For this review, take the finished solid that the model builds, in its own axes (mm). A direction names the side the tool comes from. Coordinates: 2 decimals unless noted, no trailing zeros. Write each loop counter-clockwise with the first axis right and the second up, starting at its lowest first coordinate (ties: lowest second). Pieces come first, ordered by that corner, then holes. Notation, with made-up numbers: M -12.5,28 L 14.5,28 A28 ccw 14.5,67 Z; hole C 10.5,-23 d1. An arc over 180 degrees is marked long. One line per question, with ' | ' between items.
from build123d import *

# Parameters (mm, degrees)
F0_W         = 45.3698039055
F0_H         = 13.4970545769
F1_DEPTH     = 12.7
F2_T         = -2.54
F3_T1_DEPTH  = 40.2898039055
F4_T4_DEPTH  = 35.494099833
F4_T10_DEPTH = 35.494099833


# Not quite as in the source:
# - a fillet or chamfer that OpenCascade refuses, or shapes differently, is made with other operations: its cross-section is extruded or revolved along the edge and cut away or added


with BuildPart() as f1:
    # F0 (on Top) → F1 (new body)
    with BuildSketch(Plane.XY):
        with Locations((22.6849019527, -6.7485272884)):
            Rectangle(F0_W, F0_H)
    extrude(amount=F1_DEPTH)

    # F2
    f2_openings = [f1.faces().sort_by_distance(p)[0] for p in [
        (22.684902, -6.748527, 12.7),
    ]]
    offset(amount=F2_T, openings=f2_openings)

    # F3: chamfer of 5.08 on 2 edges, made by hand

    # F3_s2 → F3_t1 (cut)
    with BuildSketch(Plane.YZ.offset(2.54)):
        Polygon((-16.0370545769, 12.7), (-10.9570545769, 7.62), (-10.9570545769, 12.7), align=None)
        Polygon((2.54, 12.7), (-2.54, 7.62), (-2.54, 12.7), align=None)
    extrude(amount=F3_T1_DEPTH, mode=Mode.SUBTRACT)

    # F4: fillet of radius 5.08 on 2 edges, made by hand


with BuildPart() as f4_tool2:
    # F4_s3 → F4_t4 (new body)
    with BuildSketch(Plane.XZ.offset(24.4955772049)):
        with BuildLine():
            ThreePointArc((45.3698039055, 12.7), (43.5103948543, 10.8405909488), (42.8298039055, 8.3005909488))
            Line((42.8298039055, 8.3005909488), (42.8298039055, 12.7))
            Line((42.8298039055, 12.7), (45.3698039055, 12.7))
        make_face()
    extrude(amount=-F4_T4_DEPTH)

    split(bisect_by=Plane(origin=(0, -1.6685272884, -1.6685272884), x_dir=(1, 0, 0), z_dir=(0, 0.7071067812, 0.7071067812)), keep=Keep.TOP)

    split(bisect_by=Plane(origin=(0, -5.08, 5.08), x_dir=(1, 0, 0), z_dir=(0, -0.7071067812, 0.7071067812)), keep=Keep.TOP)


with BuildPart() as f1_1:
    add(f1.part)

    # F4_t1: cut F4_tool2
    add(f4_tool2.part, mode=Mode.SUBTRACT)


with BuildPart() as f4_tool8:
    # F4_s9 → F4_t10 (new body)
    with BuildSketch(Plane.XZ.offset(24.4955772049)):
        with BuildLine():
            ThreePointArc((2.54, 8.3005909488), (1.8594090512, 10.8405909488), (0, 12.7))
            Line((0, 12.7), (2.54, 12.7))
            Line((2.54, 12.7), (2.54, 8.3005909488))
        make_face()
    extrude(amount=-F4_T10_DEPTH)

    split(bisect_by=Plane(origin=(0, -1.6685272884, -1.6685272884), x_dir=(1, 0, 0), z_dir=(0, 0.7071067812, 0.7071067812)), keep=Keep.TOP)

    split(bisect_by=Plane(origin=(0, -5.08, 5.08), x_dir=(1, 0, 0), z_dir=(0, -0.7071067812, 0.7071067812)), keep=Keep.TOP)


with BuildPart() as f1_2:
    add(f1_1.part)

    # F4_t7: cut F4_tool8
    add(f4_tool8.part, mode=Mode.SUBTRACT)


solid = f1_2.part
1) We need section B-B on x = 20.5. State the section outline as (y, z) points.
Responses:
outline: M -13.5,0 L 0,0 L 0,10.16 L -2.54,7.62 L -2.54,2.54 L -10.96,2.54 L -10.96,7.62 L -13.5,10.16 Z
2) To check wall thickness, follow line 1 along Y through (x, z) = (32, 7); line 2 along Z through (x, y) = (39, -10); line 3 along X through (y, z) = (-8.75, 4.75). State the ranges of each line that lie inside material, in increasing order. Write a range as [from, to].
Responses:
line 1: [-13.5, -10.96], [-2.54, 0] | line 2: [0, 2.54] | line 3: [0, 2.54], [42.83, 45.37]
3) We need section C-C on z = 10.75. State the section outline as (x, y) points, then the cut area to 3 significant figures.
Responses:
outline: M 0,-13.5 L 1.91,-13.5 L 1.91,0 L 0,0 Z; M 43.46,-13.5 L 45.37,-13.5 L 45.37,0 L 43.46,0 Z | area: 51.6 mm^2
4) Machinability: for faces 1 (the flat face through (2.54, -7, 5)), 2 (the flat face through (0, -7, 6)), which of the approach directions +Z, -Z, +X, -X, +Y, -Y give a long, thin tool a straight path to every point of the face, cutting with its end or side? Answer none if there is none.
Responses:
face 1: +Z | face 2: +Z, -Z, -X, +Y, -Y
5) The part is to be moulded in two halves that separate along X. For faces 3 (the flat face through (22.4, -1.25, 8.91)), 4 (the flat face through (45.37, -7, 6)), 5 (the flat face through (22, -13.497, 5)), say which applies: +X half, -X half, draft (parallel to the pull), parting line (faces both ways), or undercut.
Responses:
face 3: undercut | face 4: +X half | face 5: draft
6) Insertion check: pin 1 Ø1.5 at (x, y) = (32.5, -2.5) entering from +Z; pin 2 Ø2.5 at (x, y) = (26, -5) entering from +Z. Each pin has a flat end and moves straight along its axis. Give the tip position at first contact, or say it passes through.
Responses:
pin 1: z = 8.41 | pin 2: z = 2.54
7) We need section D-D on y = -3.5. State the section outline as (x, z) points, then the cut area to 3 significant figures.
Responses:
outline: M 0,0 L 45.37,0 L 45.37,12.7 A5.08 ccw 42.83,8.3 L 42.83,2.54 L 2.54,2.54 L 2.54,8.3 A5.08 ccw 0,12.7 Z | area: 160 mm^2
8) We need section A-A on z = 3.25. State the section outline as (x, y) points, then the cut area to 3 significant figures.
Responses:
outline: M 0,-13.5 L 45.37,-13.5 L 45.37,0 L 0,0 Z; hole M 2.54,-10.96 L 42.83,-10.96 L 42.83,-2.54 L 2.54,-2.54 Z | area: 273 mm^2
